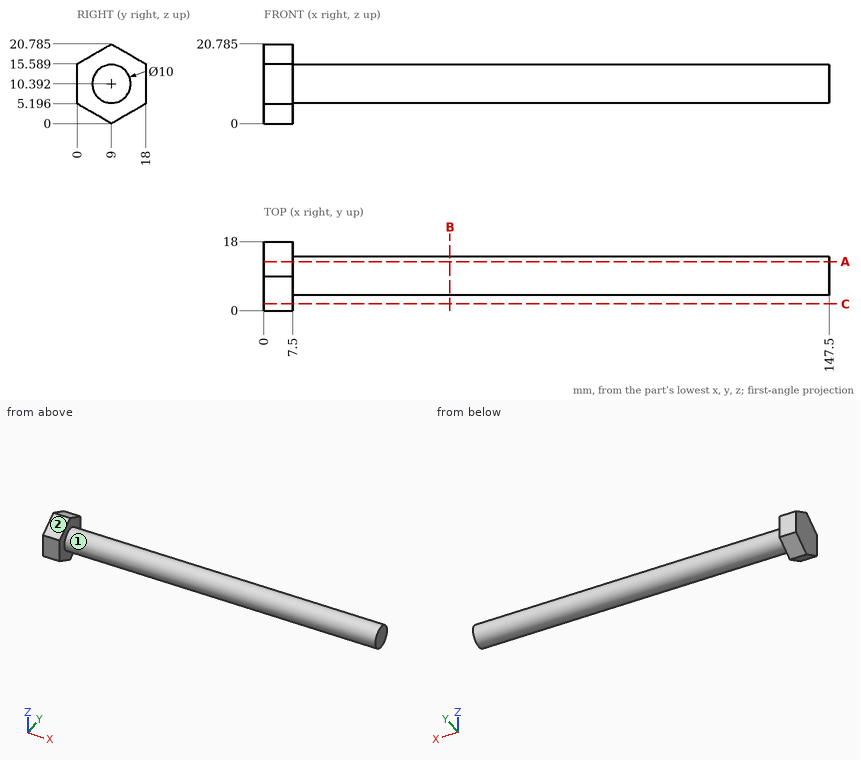
Part print with two shaded views. Sizes in mm from the minimum x, y, z corner. A direction names the side the tool comes from. Round coordinates to 2 decimals unless told otherwise and drop trailing zeros. Order: outer loops, then holes, each group sorted by start corner. A loop starts at its lowest first (then second) coordinate and runs counter-clockwise, first axis right, second up. Notation, with made-up numbers: (83.5, 4.25) - (128.5, 4.25) arc R21 cw to (128.5, 29.25) - close; hole circle Ø10 at (-33, 6.25). An arc over 180 degrees is marked (long way). Return JSON: item names as keys, results as strings.
(1) Wall check: probe 1 along X at (y, z) = (3.75, 8.75); probe 2 along Y at (x, z) = (42.5, 10.5); probe 3 along Z at (x, y) = (61, 9.5). Give the ranges that are in metal, low to high. Write a range as from..to.
Answer key:
{"probe 1": "x = 0..7.5", "probe 2": "y = 4..14", "probe 3": "z = 5.42..15.37"}
(2) Cut at B-B (x = 48.5). Give the cut face in (y, z).
Answer key:
{"outline": "circle Ø10 at (9, 10.39)"}
(3) Tool access for the marked faces 1 and 2: list every direction of +Z, -Z, +X, -X, +Y, -Y with a clear straight run to the whole face (end or side of a thin tool).
Answer key:
{"face 1": "+X", "face 2": "+Z, +X, -X, -Y"}
(4) Cut at C-C (y = 1.75). Give the cut face in (x, z) (1 decimal), then the cut area to 3 significant figures.
Answer key:
{"outline": "(0, 4.2) - (7.5, 4.2) - (7.5, 16.6) - (0, 16.6) - close", "area": "93.1 mm^2"}
(5) Pin check, flat tips, straight feed: pin 1 Ø5 at (x, y) = (131.5, 13) entering from +Z; pin 2 Ø8 at (x, z) = (76.5, 6.5) entering from -Y; pin 3 Ø2 at (x, y) = (94.5, 14) entering from +Z. Stop position of each tip, or through.
Answer key:
{"pin 1": "stops at z = 15.16", "pin 2": "stops at y = 4", "pin 3": "stops at z = 13.39"}
(6) Cut at A-A (y = 12.75). Give the cut face in (x, z) (1 decimal).
Answer key:
{"outline": "(0, 2.2) - (7.5, 2.2) - (7.5, 7.1) - (147.5, 7.1) - (147.5, 13.7) - (7.5, 13.7) - (7.5, 18.6) - (0, 18.6) - close"}
